from build123d import *

# Parameters (mm, degrees)
SKETCH1_R           = 5.5
BOSS_EXTRUDE1_DEPTH = 6


with BuildPart() as part:
    # Sketch1 → Boss-Extrude1 (new body)
    with BuildSketch(Plane(origin=(0, 0, 0), x_dir=(1, 0, 0), z_dir=(0, 1, 0))):
        with BuildLine():
            Line((7.5, 8.602325267), (7.5, 13.602325267))
            Line((7.5, 13.602325267), (4.9, 13.602325267))
            Line((4.9, 13.602325267), (4.9, 19.102325267))
            Line((4.9, 19.102325267), (-4.9, 19.102325267))
            Line((-4.9, 19.102325267), (-4.9, 13.602325267))
            Line((-4.9, 13.602325267), (-7.5, 13.602325267))
            Line((-7.5, 13.602325267), (-7.5, 8.602325267))
            ThreePointArc((-7.5, 8.602325267), (-7.75978466, 6.337771199), (-8.525641026, 4.190876412))
            ThreePointArc((-8.525641026, 4.190876412), (0, -9.5), (8.525641026, 4.190876412))
            ThreePointArc((8.525641026, 4.190876412), (7.75978466, 6.337771199), (7.5, 8.602325267))
        make_face()
        with Locations(Location((0, 0, 0), (0, 0, 270))):
            Circle(SKETCH1_R, mode=Mode.SUBTRACT)
    extrude(amount=BOSS_EXTRUDE1_DEPTH)


solid = part.part
Model file for the job. Use its own axes, mm. A direction names the side the tool comes from. Give positions to 0.01 mm unless a question says otherwise; leave off trailing zeros. Write each loop counter-clockwise with the first axis right and the second up, starting at its lowest first coordinate (ties: lowest second). Pieces come first, ordered by that corner, then holes. Notation, with made-up numbers: M 65,-39 L 121,-39 A24 ccw 121,-7 Z; hole C 35,29 d4. An arc over 180 degrees is marked long. One line per item, written item: value. Start each with the question number.
Q1. Saw through at D-D, the plane z = -10.5. Write the cut outline in (x, y), plus the area to 3 significant figures.
Q2. Saw through at C-C, the plane z = 0. Write the cut outline in (x, y), plus the area to 3 significant figures.
Q3. Saw through at A-A, the plane x = 0. Write the cut outline in (y, z), plus the area to 3 significant figures.
Q4. Two-plate mould, pull along Z, no slides. Class faces 1 (the flat face through (0, 6, -8)), 2 (the cylindrical face through (7.767, 2.958, -6.307)), 3 (the cylindrical face through (-5.37, 2.96, -1.19)): +Z half, -Z half, draft (parallel to the pull), parting line (faces both ways), or undercut.
Q5. Probe probe 1 along X at (y, z) = (3.3, 0); probe 2 along X at (y, z) = (1.15, -13.25); probe 3 along X at (y, z) = (4.4, 2). List the from-to ranges inside material, lowest first. Write a range as [from, to].
Q6. Drop flat-ended pins along their axis: pin 1 Ø2.5 at (y, z) = (2.5, -10) entering from -X; pin 2 Ø1.7 at (y, z) = (3.5, -16) entering from -X; pin 3 Ø1 at (x, y) = (2, 2) entering from +Z. Give the stop position or say it passes through.
Q7. Saw through at B-B, the plane y = 4.75. Write the cut outline in (x, z), plus the area to 3 significant figures.
Q8. 3-axis set-ups, long thin cutter, end or side, ignore diameter. For faces 4 (the flat face through (0, 3, -19.102)), 5 (the flat face through (-4.9, 3, -16)), 6 (the flat face through (4.9, 3, -16)): which of +Z, -Z, +X, -X, +Y, -Y reach the whole face in a straight line?
Output values:
1. outline: M -7.5,0 L 7.5,0 L 7.5,6 L -7.5,6 Z
1. area: 90.0 mm²
2. outline: M -9.5,0 L -5.5,0 L -5.5,6 L -9.5,6 Z; M 5.5,0 L 9.5,0 L 9.5,6 L 5.5,6 Z
2. area: 48.0 mm²
3. outline: M 0,-19.1 L 6,-19.1 L 6,-5.5 L 0,-5.5 Z; M 0,5.5 L 6,5.5 L 6,9.5 L 0,9.5 Z
3. area: 106 mm²
4. face 1: draft
4. face 2: -Z half
4. face 3: undercut
5. probe 1: x = [-9.5, -5.5], [5.5, 9.5]
5. probe 2: x = [-7.5, 7.5]
5. probe 3: x = [-9.29, -5.12], [5.12, 9.29]
6. pin 1: stops at x = -7.5
6. pin 2: stops at x = -4.9
6. pin 3: stops at z = 9.38
7. outline: M -8.53,-4.19 A10 cw -7.5,-8.6 L -7.5,-13.6 L -4.9,-13.6 L -4.9,-19.1 L 4.9,-19.1 L 4.9,-13.6 L 7.5,-13.6 L 7.5,-8.6 A10 cw 8.53,-4.19 A9.5 ccw long Z; hole C 0,0 d11
7. area: 322 mm²
8. face 4: -Z, +X, -X, +Y, -Y
8. face 5: -Z, -X, +Y, -Y
8. face 6: -Z, +X, +Y, -Y
